Verification items for the finished model (mm, model axes). Face numbers are marked on the shaded views. A direction names the side the tool comes from. Round coordinates to 2 decimals unless told otherwise and drop trailing zeros. Write each loop counter-clockwise with the first axis right and the second up, starting at its lowest first coordinate (ties: lowest second). Pieces come first, ordered by that corner, then holes. Notation, with made-up numbers: (34, 50.25) - (39, 50.25) arc R21 cw to (39, 87.25) - close; hole circle Ø9 at (56.5, 43). An arc over 180 degrees is marked (long way). Write each question's results on one line, items separated by ' | '.
Autodesk Inventor part; units mm, degrees
ref_plane "XZ Plane" through (0, 0, 0) normal (0, 1, 0) x (-1, 0, 0)
ref_plane "XY Plane" through (0, 0, 0) normal (0, 0, 1) x (1, 0, 0)
ref_plane "Work Plane1" through (0, 0, -3.25) normal (0, 0, -1) x (-1, 0, 0)
sketch "Sketch1" plane through (0, 0, 0) normal (0, 0, 1) x (1, 0, 0)
  line L0 (-27.5, 6.775) -> (27.5, 6.775)
  line L1 (27.5, 6.775) -> (27.5, -5.925)
  line L2 (27.5, -5.925) -> (-27.5, -5.925)
  line L3 (-27.5, -5.925) -> (-27.5, 6.775)
  point P0 (0, 0)
  dimension "d0" = 6.775
  dimension "d1" = 5.925
  dimension "d2" = 27.5
  dimension "d3" = 27.5
extrude "Extrusion1" add sketch "Sketch1" along normal blind 10
ref_plane "Work Plane1" through (0, 0, -3.25) normal (0, 0, -1) x (-1, 0, 0)
sketch "Sketch2" plane through (0, 0, -3.25) normal (0, 0, -1) x (-1, 0, 0)
  line L0 (27.5, 6.775) -> (-27.5, 6.775)
  line L1 (-27.5, -5.925) -> (27.5, -5.925)
  line L2 (0, 6.775) -> (-8.1, 6.775)
  line L3 (-27.5, 6.775) -> (27.5, 6.775)
  line L4 (-8.1, 6.775) -> (-8.1, 2.825)
  line L5 (-8.1, 2.825) -> (-6.25, 2.825)
  line L6 (-6.25, 2.825) -> (-6.25, -2.825)
  line L7 (-6.25, -2.825) -> (-8.1, -2.825)
  line L8 (-8.1, -2.825) -> (-8.1, -5.925)
  line L9 (27.5, -5.925) -> (-27.5, -5.925)
  line L10 (-8.1, -5.925) -> (0, -5.925)
  line L11 (0, -5.925) -> (0, 6.775)
  line L12 (0, -8.465) -> (0, 9.315)
  point P0 (0, 0)
  dimension "d7" = 8.1
  dimension "d8" = 6.25
  dimension "d9" = 3.95
  dimension "d10" = 3.1
revolve "Revolution1" cut sketch "Sketch2" angle 180 about axis through (0, 0, -3.25) along (0, -1, 0)
sketch "Sketch3" plane through (0, 0, 10) normal (0, 0, 1) x (1, 0, 0)
  line L0 (0, 0) -> (43.2339, 0) construction
  line L1 (0, 0) -> (-39.8542, 0) construction
  point P0 (-12.5, 0)
  point P1 (12.5, 0)
  dimension "d12" = 12.5
  dimension "d13" = 12.5
hole "Hole1" at (-12.5, 0, 10) at (12.5, 0, 10) direction (0, 0, -1) diameter 3.5 end through all counterbore diameter 6.5 counterbore depth 3
sketch "Sketch5" plane through (-27.5, 6.775, 10) normal (0, 1, 0) x (1, 0, 0)
  arc A0 (22.1615, 10) -> (32.8385, 10) centre (27.5, 13.25) ccw
  line L0 (27.5, 13.25) -> (61.0026, 13.25) construction
  line L1 (55, 10) -> (55, 0)
  circle A1 centre (49, 13.25) radius 5
  point P0 (27.5, 10)
  dimension "d26" = 6
  dimension "d27" = 10
extrude "Extrusion3" cut sketch "Sketch5" against normal through all
sketch "Sketch6" plane through (-12.5, 0, 7) normal (0, 0, 1) x (1, 0, 0)
  circle A0 centre (0, 0) radius 1.75
  circle A1 centre (25, 0) radius 1.75
  point P0 (12.5, 0)
extrude "Extrusion4" add sketch "Sketch6" against normal blind 0.4
fillet "Fillet2" radius 1 4 edges at (-27.5, 6.775, 5) (-27.5, -5.925, 5) (27.5, 6.775, 5) (27.5, -5.925, 5)
properties part number "Retainer_10mm" material "PC/ABS Plastic"
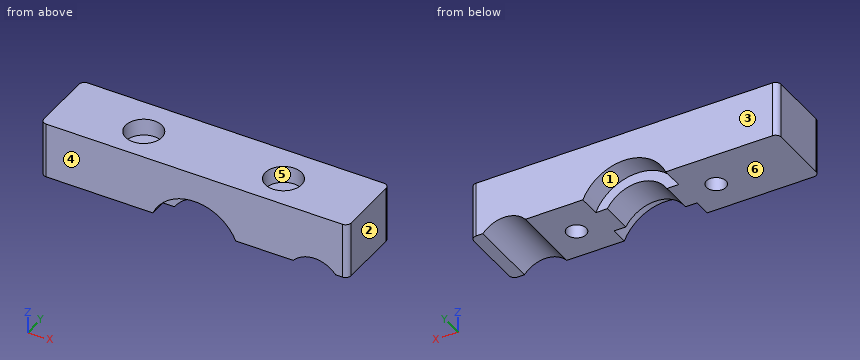
(1) Thickness scan on L1, parallel to X at y = 0, z = 4; L2, parallel to X at y = 0, z = 7.95; L3, parallel to Y at x = 12.5, z = 4.75 (3 decimals). Record the ranges inside material, lowest first.
Answer:
L1: -27.5 to -14.25, -10.75 to 10.75, 14.25 to 27.5 | L2: -27.5 to -15.75, -9.25 to 9.25, 15.75 to 27.5 | L3: -5.925 to -1.75, 1.75 to 6.775
(2) Section check B-B (z = 8.25). Record the cut outline in (x, y) (3 decimals), plus the area to 3 significant figures.
Answer:
outline: (-27.5, -4.925) arc R1 ccw to (-26.5, -5.925) - (26.5, -5.925) arc R1 ccw to (27.5, -4.925) - (27.5, 5.775) arc R1 ccw to (26.5, 6.775) - (-26.5, 6.775) arc R1 ccw to (-27.5, 5.775) - close; hole circle Ø6.5 at (-12.5, 0); hole circle Ø6.5 at (12.5, 0) | area: 631 mm2
(3) Go/stop test with flat-tipped pins: pin 1 Ø4 at (x, z) = (-1.5, 1.5) entering from +Y (3 decimals); pin 2 Ø1 at (x, y) = (-12, 0) entering from -Z; pin 3 Ø3 at (x, y) = (13, -1) entering from +Z. Record where each tip stops, or that it passes through.
Answer:
pin 1: y = 2.825 | pin 2: z = 6.6 | pin 3: z = 7
(4) Mould release check, pull along Y, two halves, no side actions. Record for the marked faces 3, 4, 5 and 6: released by +Y, released by -Y, zero draft, split by the parting line, or undercut.
Answer:
face 3: released by +Y | face 4: released by -Y | face 5: undercut | face 6: zero draft
(5) Section check A-A (y = 4.75). Record the cut outline in (x, z), plus the area to 3 significant figures.
Answer:
outline: (-27.5, 0) - (-7.42, 0) arc R8.1 cw to (7.42, 0) - (17.7, 0) arc R5 cw to (25.3, 0) - (27.5, 0) - (27.5, 10) - (-27.5, 10) - close | area: 489 mm2
(6) Set-up check for the marked faces 1 and 2: record each of +Z, -Z, +X, -X, +Y, -Y from which the full face is reachable in a straight line by a thin tool's end or side.
Answer:
face 1: -Z, +Y | face 2: +Z, -Z, +X, +Y, -Y
(7) Section check D-D (x = 0). Record the cut outline in (y, z) (3 decimals).
Answer:
outline: (-5.925, 4.85) - (-2.825, 4.85) - (-2.825, 3) - (2.825, 3) - (2.825, 4.85) - (6.775, 4.85) - (6.775, 10) - (-5.925, 10) - close
(8) Section check C-C (x = -12.5). Record the cut outline in (y, z) (3 decimals), plus the area to 3 significant figures.
Answer:
outline: (-5.925, 0) - (-1.75, 0) - (-1.75, 6.6) - (1.75, 6.6) - (1.75, 0) - (6.775, 0) - (6.775, 10) - (3.25, 10) - (3.25, 7) - (-3.25, 7) - (-3.25, 10) - (-5.925, 10) - close | area: 84.4 mm2
